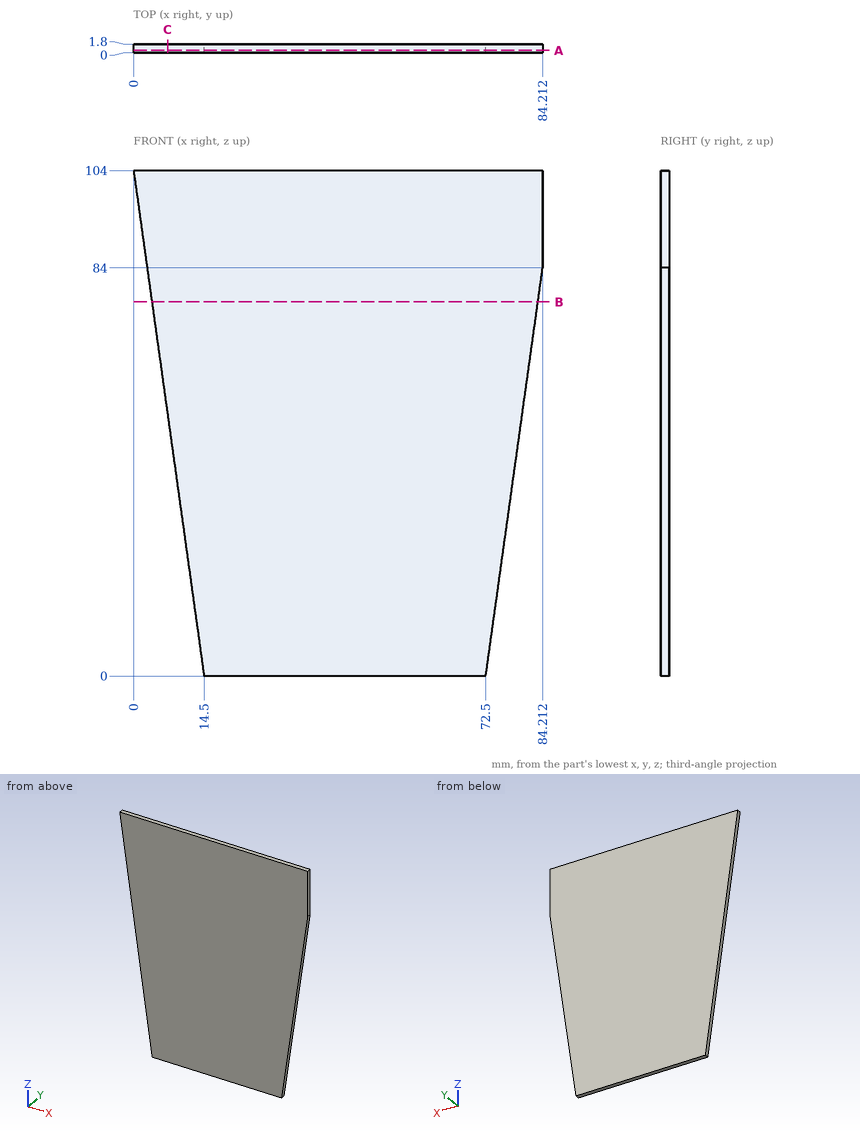
Geometry: see drawing. Coordinates: mm, zero at the bounding-box minimum. Give positions to 0.01 mm unless a question says otherwise; leave off trailing zeros. Write each loop counter-clockwise with the first axis right and the second up, starting at its lowest first coordinate (ties: lowest second). Pieces come first, ordered by that corner, then holes. Notation, with made-up numbers: M 69.25,72.5 L 82.25,72.5 A17 ccw 82.25,88.5 Z; hole C 18,-28 d7. An arc over 180 degrees is marked long. Return JSON: item names as keys, results as strings. Group by question number.
1) First-contact query: pin 1 Ø2 at (x, z) = (29.5, 64.5) entering from -Y. Flat tip, straight axial feed; report the tip coordinate or a pass-through.
2) Cut plane B-B, the plane z = 77. Output: boundary loops of the cut face in (x, y) (1 decimal).
3) Cut plane A-A, the plane y = 0.5. Output: boundary loops of the cut face in (x, z).
4) Ray query, L1, parallel to X at y = 0.15, z = 91; L2, parallel to X at y = 0.75, z = 14.5. Return the intervals inside material, ascending.
5) Cut plane C-C, the plane x = 7. Output: boundary loops of the cut face in (y, z).
Data:
{
 "1": {"pin 1": "stops at y = 0"},
 "2": {"outline": "M 3.8,0 L 83.2,0 L 83.2,1.8 L 3.8,1.8 Z"},
 "3": {"outline": "M 0,104 L 14.5,0 L 72.5,0 L 84.21,84 L 84.21,104 Z"},
 "4": {"L1": "x = 1.81 to 84.21", "L2": "x = 12.48 to 74.52"},
 "5": {"outline": "M 0,53.79 L 1.8,53.79 L 1.8,104 L 0,104 Z"}
}
